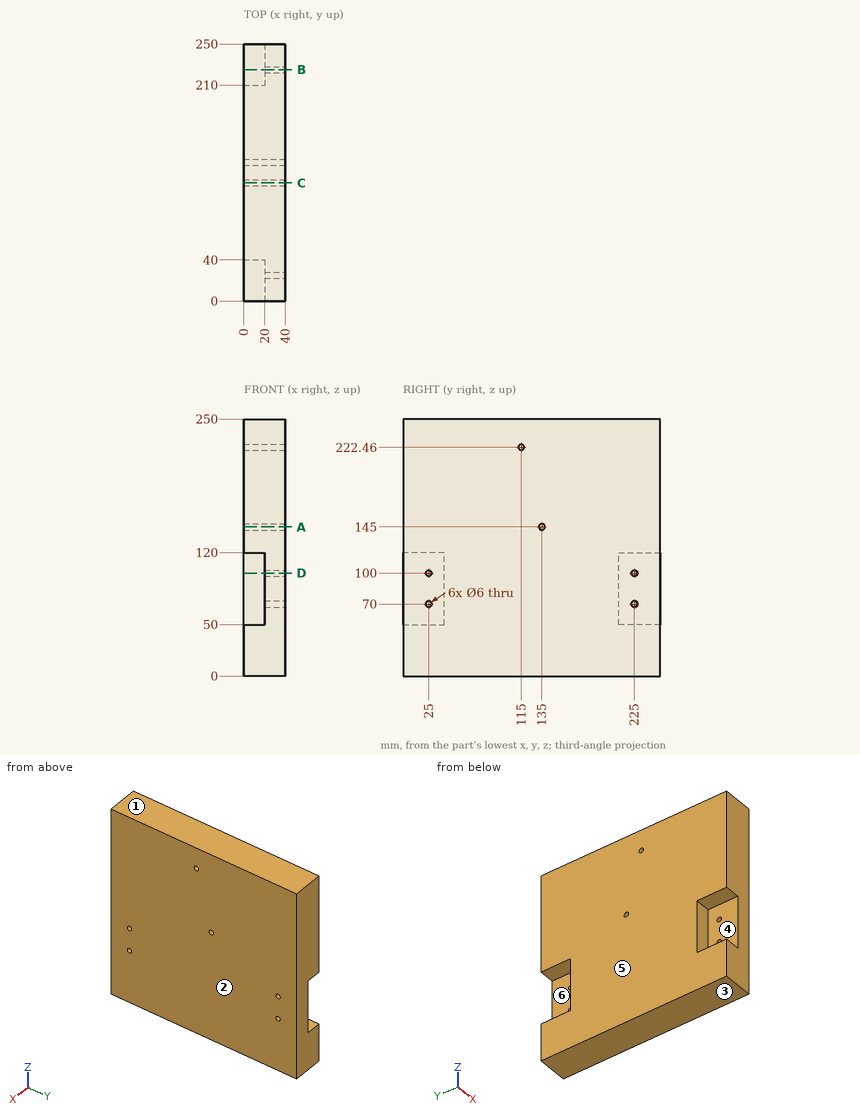
Verification items for this drawing (mm, ordinates from the low corner). A direction names the side the tool comes from. Give positions to 0.01 mm unless a question says otherwise; leave off trailing zeros. Loops run counter-clockwise (first coordinate to the right, second up) from the corner with the lowest first, then second, coordinate; pieces in that order, holes last. Notation, with made-up numbers: M -21,58.5 L 24,58.5 A4 ccw 24,63.5 Z; hole C 13,85.25 d3. An arc over 180 degrees is marked long. Write item = value, one per line. Start each with the question number.
1. Section check A-A, the plane z = 145. Enter the section's corners in (x, y), plus the area to 3 significant figures.
2. Section check C-C, the plane y = 115. Enter the section's corners in (x, z), plus the area to 3 significant figures.
3. Draft check along Z on the marked faces 1, 2, 3 and 4. Enter one of: +Z half, -Z half, draft (parallel to the pull), parting line (faces both ways), or undercut.
4. Thickness scan on probe 1 along Y at (x, z) = (35, 100); probe 2 along Z at (x, y) = (27.5, 25); probe 3 along Z at (x, y) = (26, 115). Record the ranges inside material, lowest first.
5. Section check D-D, the plane z = 100. Enter the section's corners in (x, y).
6. Tool access check on the marked faces 5 and 6. Record the directions out of +Z, -Z, +X, -X, +Y, -Y that give a thin tool (end or side, any length) a straight path to the whole face; none if there is none.
7. Section check B-B, the plane y = 225. Enter the section's corners in (x, z), plus the area to 3 significant figures.
8. Go/stop test with flat-tipped pins: P1, Ø20, axis at y = 237.5, z = 101.5, coming from the -X side; P2, Ø10, axis at x = 7, z = 69, coming from the +Y side; P3, Ø3.5, axis at y = 25, z = 100, coming from the +X side; P4, Ø10, axis at x = 10.5, z = 75.5, coming from the -Y side. Record where each tip stops, or that it passes through.
Values follow:
q1.outline = M 0,0 L 40,0 L 40,132 L 0,132 Z; M 0,138 L 40,138 L 40,250 L 0,250 Z
q1.area = 9,760 mm^2
q2.outline = M 0,0 L 40,0 L 40,219.46 L 0,219.46 Z; M 0,225.46 L 40,225.46 L 40,250 L 0,250 Z
q2.area = 9,760 mm^2
q3.face_1 = +Z half
q3.face_2 = draft
q3.face_3 = -Z half
q3.face_4 = undercut
q4.probe_1 = 0 to 22, 28 to 222, 228 to 250
q4.probe_2 = 0 to 67, 73 to 97, 103 to 250
q4.probe_3 = 0 to 219.46, 225.46 to 250
q5.outline = M 0,40 L 20,40 L 20,28 L 40,28 L 40,222 L 20,222 L 20,210 L 0,210 Z; M 20,0 L 40,0 L 40,22 L 20,22 Z; M 20,228 L 40,228 L 40,250 L 20,250 Z
q6.face_5 = +Z, -Z, -X, +Y, -Y
q6.face_6 = -X, +Y
q7.outline = M 0,0 L 40,0 L 40,67 L 20,67 L 20,50 L 0,50 Z; M 0,120 L 20,120 L 20,103 L 40,103 L 40,250 L 0,250 Z; M 20,73 L 40,73 L 40,97 L 20,97 Z
q7.area = 8,360 mm^2
q8.P1 = 20
q8.P2 = 210
q8.P3 = through
q8.P4 = 40
